from build123d import *

# Parameters (mm, degrees)
SKETCH1_W                      = 158
SKETCH1_H                      = 199.5
BOSS_EXTRUDE1_DEPTH            = 6.35
BOSS_EXTRUDE2_DEPTH            = 12.7
CBORE_FOR_M4_SHCS1_D           = 4.5
CBORE_FOR_M4_SHCS1_DEPTH       = 6.35
CBORE_FOR_M4_SHCS1_CBORE_D     = 8
CBORE_FOR_M4_SHCS1_CBORE_DEPTH = 4
FILLET2_R                      = 5
SKETCH8_R                      = 3
ENCLOSURE_MOUNT_DEPTH          = 7.35
SKETCH9_R                      = 2.5
FUSE_MOUNT_DEPTH               = 7.35
SKETCH10_R                     = 3.05
MAGNETS_DEPTH                  = 3.1


with BuildPart() as part:
    # Sketch1 → Boss-Extrude1 (new body)
    with BuildSketch(Plane(origin=(0, 0, 0), x_dir=(1, 0, 0), z_dir=(0, 1, 0))):
        with Locations((79, -99.75)):
            Rectangle(SKETCH1_W, SKETCH1_H)
    extrude(amount=BOSS_EXTRUDE1_DEPTH)

    # Sketch3 → Boss-Extrude2 (add)
    with BuildSketch(Plane(origin=(0, 6.35, 0), x_dir=(1, 0, 0), z_dir=(0, 1, 0))):
        Polygon((0, 0), (0, -199.5), (158, -199.5), (158, -194.5), (5, -194.5), (5, 0), align=None)
    extrude(amount=BOSS_EXTRUDE2_DEPTH)

    # CBORE for M4 SHCS1
    with Locations(Plane(origin=(0, 6.35, 0), x_dir=(1, 0, 0), z_dir=(0, 1, 0))):
        with Locations((20, -55), (98, -179.5), (138, -179.5), (20, -130), (20, -105), (20, -30)):
            CounterBoreHole(CBORE_FOR_M4_SHCS1_D / 2, CBORE_FOR_M4_SHCS1_CBORE_D / 2, CBORE_FOR_M4_SHCS1_CBORE_DEPTH, depth=CBORE_FOR_M4_SHCS1_DEPTH)

    # Fillet2
    fillet2_edges = [part.edges().sort_by_distance(p)[0] for p in [
        (5, 12.7, 194.5),
        (0, 9.525, 199.5),
    ]]
    fillet(fillet2_edges, radius=FILLET2_R)

    # Sketch8 → Enclosure Mount (cut, through all)
    with BuildSketch(Plane(origin=(0, 6.35, 0), x_dir=(1, 0, 0), z_dir=(0, 1, 0))):
        with Locations((46.1, -52.5)):
            Circle(SKETCH8_R)
        with Locations((122.3, -52.5)):
            Circle(SKETCH8_R)
        with Locations((122.3, -179.5)):
            Circle(SKETCH8_R)
        with Locations((46.1, -179.5)):
            Circle(SKETCH8_R)
    extrude(amount=-ENCLOSURE_MOUNT_DEPTH, mode=Mode.SUBTRACT)

    # Sketch9 → Fuse Mount (cut, through all)
    with BuildSketch(Plane(origin=(0, 6.35, 0), x_dir=(1, 0, 0), z_dir=(0, 1, 0))):
        with Locations((11.75, -15)):
            Circle(SKETCH9_R)
        with Locations((151.25, -15)):
            Circle(SKETCH9_R)
    extrude(amount=-FUSE_MOUNT_DEPTH, mode=Mode.SUBTRACT)

    # Sketch10 → Magnets (cut)
    with BuildSketch(Plane(origin=(0, 6.35, 0), x_dir=(1, 0, 0), z_dir=(0, 1, 0))):
        with Locations((151.25, -34.9)):
            Circle(SKETCH10_R)
        with Locations((73.375, -34.9)):
            Circle(SKETCH10_R)
    extrude(amount=-MAGNETS_DEPTH, mode=Mode.SUBTRACT)


solid = part.part
Can you work these out from the model? Positions are in its coordinate system, mm. A direction names the side the tool comes from. Coordinates: 2 decimals unless noted, no trailing zeros. Loops run counter-clockwise (first coordinate to the right, second up) from the corner with the lowest first, then second, coordinate; pieces in that order, holes last. Notation, with made-up numbers: M -34,14.5 L 25,14.5 A36 cw 25,49.5 Z; hole C -25,64 d7. An arc over 180 degrees is marked long. Return JSON: item names as keys, results as strings. Group by question number.
Item 1: Imagine slicing it at A-A (x = 122.3). Please give me the cut outline in (y, z).
Item 2: On a 3-axis mill with a long thin cutter (end or side, diameter ignored), from which of +Z, -Z, +X, -X, +Y, -Y can I reach the whole of each face in a straight line? I mean faces 4 (the cylindrical face through (96.962, 1.159, 181.496)), 5 (the cylindrical face through (21.846, 4.378, 108.549)), 6 (the flat face through (80, 6.35, 96)). Say none if no direction works.
Item 3: Thinking about a two-plate mould opening in X: for faces 1 (the cylindrical face through (45.709, 3.219, 49.526)), 2 (the cylindrical face through (1.43, 9.66, 198)), 3 (the cylindrical face through (6.43, 12.79, 193)), which applies, released by +X, released by -X, zero draft, split by the parting line, or undercut?
Item 4: Imagine slicing it at B-B (y = 9.75). Please give me the cut outline in (x, z), and give its area (3 significant figures).
Item 5: I'm going to push flat-ended pins straight in: pin 1 Ø7 at (x, z) = (20, 130) entering from +Y; pin 2 Ø1 at (x, z) = (108, 171) entering from -Y; pin 3 Ø6.5 at (y, z) = (11, 110) entering from +X; pin 4 Ø2 at (x, z) = (40.5, 159) entering from +Y. Where does each tip first touch, or does it pass through?
Item 6: If I drill on L1, parallel to Z at x = 20, y = 5.25; L2, parallel to X at y = 4, z = 15; L3, parallel to Z at x = 122.3, y = 2.5, over which ranges is the centre line in solid material (lowest first)? Write a range as from..to.
Item 7: Imagine slicing it at C-C (z = 105). Please give me the cut outline in (x, y), and give its area (3 significant figures).
Item 8: Imagine slicing it at D-D (x = 20). Give the number of separate pieces and of enclosed holes in the cut face, and give its area (3 significant figures).
Verdict:
{
 "1": {"outline": "M 0,0 L 6.35,0 L 6.35,49.5 L 0,49.5 Z; M 0,55.5 L 6.35,55.5 L 6.35,176.5 L 0,176.5 Z; M 0,182.5 L 6.35,182.5 L 6.35,194.5 L 19.05,194.5 L 19.05,199.5 L 0,199.5 Z"},
 "2": {"face 4": "+Y, -Y", "face 5": "+Y", "face 6": "-Z, +X, +Y"},
 "3": {"face 1": "undercut", "face 2": "released by -X", "face 3": "released by +X"},
 "4": {"outline": "M 0,0 L 5,0 L 5,189.5 A5 cw 10,194.5 L 158,194.5 L 158,199.5 L 5,199.5 A5 ccw 0,194.5 Z", "area": "1,760 mm^2"},
 "5": {"pin 1": "stops at y = 2.35", "pin 2": "stops at y = 0", "pin 3": "stops at x = 5", "pin 4": "stops at y = 6.35"},
 "6": {"L1": "z = 0..26, 34..51, 59..101, 109..126, 134..199.5", "L2": "x = 0..9.25, 14.25..148.75, 153.75..158", "L3": "z = 0..49.5, 55.5..176.5, 182.5..199.5"},
 "7": {"outline": "M 0,0 L 17.75,0 L 17.75,2.35 L 16,2.35 L 16,6.35 L 5,6.35 L 5,19.05 L 0,19.05 Z; M 22.25,0 L 158,0 L 158,6.35 L 24,6.35 L 24,2.35 L 22.25,2.35 Z", "area": "1,020 mm^2"},
 "8": {"separate pieces": "5", "enclosed holes": "0", "area": "1,160 mm^2"}
}
